```python
from build123d import *

# Parameters (mm, degrees)
F1_DEPTH = 35


with BuildPart() as f1:
    # F0 (on Top) → F1 (new body)
    with BuildSketch(Plane.XY):
        with BuildLine():
            Line((9, 17.5), (-9, 17.5))
            ThreePointArc((-9, 17.5), (-12.889087, 15.889087), (-14.5, 12))
            Line((-14.5, 12), (-14.5, -3.481193))
            ThreePointArc((-14.5, -3.481193), (-12.057349, -14.131547), (-1.2669, -12.410275))
            ThreePointArc((-1.2669, -12.410275), (-0.082689, -11.830952), (1.101521, -12.410275))
            ThreePointArc((1.101521, -12.410275), (11.749259, -14.225639), (14.5, -3.780388))
            Line((14.5, -3.780388), (14.5, 12))
            ThreePointArc((14.5, 12), (12.889087, 15.889087), (9, 17.5))
        make_face()
    extrude(amount=F1_DEPTH)


solid = f1.part
```
Can you work these out from the model? Positions are in its coordinate system, mm. A direction names the side the tool comes from. Coordinates: 2 decimals unless noted, no trailing zeros. Order: outer loops, then holes, each group sorted by start corner. A loop starts at its lowest first (then second) coordinate and runs counter-clockwise, first axis right, second up.
1. If we section it at C-C (x = 3): Please give me the cut outline in (y, z), then the cut area to 3 significant figures.
2. I need wall thicknesses on line 1 (Y direction, x = -7.5, z = 20.5); line 2 (X direction, y = 3, z = 5); line 3 (Y direction, x = -13.5, z = 30). Which ranges of each line are inside material? Lowest first, please.
3. Thinking about a two-plate mould opening in X: for faces 1 (the face through (12.93, 15.85, 17.26)), 2 (the face through (-14.5, 4, 17)), 3 (the face through (0, 1, 0)), 4 (the face through (-12.196, -14.036, 17.255)), which applies, +X half, -X half, draft (parallel to the pull), parting line (faces both ways), or undercut?
4. If we section it at B-B (y = -2.5): Please give me the cut outline in (x, z), then the cut area to 4 significant figures.
5. I'm going to push flat-ended pins straight in: pin 1 (17 mm diameter, centred on y = 5.5, z = 15.5, fed in from -X); pin 2 (5 mm diameter, centred on x = 3, z = 29, fed in from -Y); pin 3 (1.5 mm diameter, centred on x = 0, z = 8, fed in from -Y). Where does each tip first touch, or does it pass through?
6. If we section it at A-A (z = 10.5): Please give me the cut outline in (x, y).
7. For faces 5 (the face through (14.5, 4, 17)), 6 (the face through (0, 17.5, 17)), which set-ups out of +Z, -Z, +X, -X, +Y, -Y let a thin tool reach every point of the face, with its end or its side?
Entries:
1. outline: (-14.17, 0) - (17.5, 0) - (17.5, 35) - (-14.17, 35) - close
1. area: 1,110 mm2
2. line 1: y = -15.5 to 17.5
2. line 2: x = -14.5 to 14.5
2. line 3: y = -12.88 to 15.16
3. face 1: +X half
3. face 2: -X half
3. face 3: draft
3. face 4: undercut
4. outline: (-14.5, 0) - (14.5, 0) - (14.5, 35) - (-14.5, 35) - close
4. area: 1,015 mm2
5. pin 1: stops at x = -14.5
5. pin 2: stops at y = -15.27
5. pin 3: stops at y = -12.08
6. outline: (-14.5, -3.48) arc R8 ccw to (-1.27, -12.41) arc R1.5 cw to (1.1, -12.41) arc R8 ccw to (14.5, -3.78) - (14.5, 12) arc R5.5 ccw to (9, 17.5) - (-9, 17.5) arc R5.5 ccw to (-14.5, 12) - close
7. face 5: +Z, -Z, +X, +Y
7. face 6: +Z, -Z, +X, -X, +Y
